Model file for the job. Use its own axes, mm. A direction names the side the tool comes from. Round coordinates to 2 decimals unless told otherwise and drop trailing zeros. Order: outer loops, then holes, each group sorted by start corner. A loop starts at its lowest first (then second) coordinate and runs counter-clockwise, first axis right, second up. Notation, with made-up numbers: (65, 17.5) -> (70, 17.5) arc R15 cw to (70, 44.5) -> close; hole circle Ø5 at (59.25, 48.25). An arc over 180 degrees is marked (long way). Use CSV: the item, a comma, the result in double quotes.
```python
from build123d import *

# Parameters (mm, degrees)
F0_R     = 12.5
F1_DEPTH = 11
F2_R     = 11.5
F3_DEPTH = 9
F4_R     = 2


with BuildPart() as f1:
    # F0 (on Top) → F1 (new body)
    with BuildSketch(Plane.XY):
        Circle(F0_R)
    extrude(amount=F1_DEPTH)

    # F2 (on face) → F3 (cut)
    with BuildSketch(Plane.XY.offset(11)):
        Circle(F2_R)
    extrude(amount=-F3_DEPTH, mode=Mode.SUBTRACT)

    # F4
    f4_edges = [f1.edges().sort_by_distance(p)[0] for p in [
        (-12.5, 0, 0),
    ]]
    fillet(f4_edges, radius=F4_R)


solid = f1.part
```
Q1. Cut at D-D (z = 1). Give the cut face in (x, y), plus the area to 3 significant figures.
From the geometry:
outline,"circle Ø24.46 at (0, 0)"
area,"470 mm²"
Q2. Which spindle directions (+Z, -Z, +X, -X, +Y, -Y) get a long thin tool onto all of the face, cutting with end or side? Do faces 4 (the flat face through (11, -4, 11)), 5 (the flat face through (0, 0, 2)). Say none if no direction does.
From the geometry:
face 4,"+Z, +X, -X, +Y, -Y"
face 5,"+Z"
Q3. Cut at C-C (z = 4). Give the cut face in (x, y), plus the area to 3 significant figures.
From the geometry:
outline,"circle Ø25 at (0, 0); hole circle Ø23 at (0, 0)"
area,"75.4 mm²"
Q4. Probe line 1 along Y through (x, z) = (0, 7.5); line 2 along Z through (x, y) = (2, -0.25); line 3 along X through (y, z) = (-4.25, 7.5). List the from-to ranges inside material, lowest first.
From the geometry:
line 1,"y = -12.5 to -11.5, 11.5 to 12.5"
line 2,"z = 0 to 2"
line 3,"x = -11.76 to -10.69, 10.69 to 11.76"
Q5. Cut at A-A (x = 0). Give the cut face in (y, z).
From the geometry:
outline,"(-12.5, 2) arc R2 ccw to (-10.5, 0) -> (10.5, 0) arc R2 ccw to (12.5, 2) -> (12.5, 11) -> (11.5, 11) -> (11.5, 2) -> (-11.5, 2) -> (-11.5, 11) -> (-12.5, 11) -> close"
Q6. Pin check, flat tips, straight feed: pin 1 (2 mm diameter, centred on x = 7.5, z = 6.5, fed in from -Y); pin 2 (4 mm diameter, centred on y = -1.5, z = 3, fed in from +X); pin 3 (1.5 mm diameter, centred on x = 5.5, y = -7, fed in from +Z); pin 4 (1.5 mm diameter, centred on x = 8.5, z = 6, fed in from +Y). Stop position of each tip, or through.
From the geometry:
pin 1,"stops at y = -10.68"
pin 2,"stops at x = 12.5"
pin 3,"stops at z = 2"
pin 4,"stops at y = 9.81"
Q7. Mould opens along X. For faces 1 (the flat face through (0, 0, 0)), 2 (the cylindrical face through (-1.5, 11.4, 6.6)), 3 (the cylindrical face through (11.923, 3.755, 6.437)) say: +X half, -X half, draft (parallel to the pull), parting line (faces both ways), or undercut.
From the geometry:
face 1,"draft"
face 2,"undercut"
face 3,"parting line"
